Autodesk Inventor part; units mm, degrees
ref_plane "YZ Plane" through (0, 0, 0) normal (1, 0, 0) x (0, 1, 0)
ref_plane "XZ Plane" through (0, 0, 0) normal (0, 1, 0) x (-1, 0, 0)
ref_plane "XY Plane" through (0, 0, 0) normal (0, 0, 1) x (1, 0, 0)
sketch "Sketch1" plane through (0, 0, 0) normal (0, 1, 0) x (-1, 0, 0)
  circle A0 centre (0, 0) radius 26
  dimension "d0" = 52
extrude "Extrusion1" add sketch "Sketch1" along normal blind 7.2
chamfer "Chamfer2" distance 2 angle 45 1 edges at (26, 0, 0)
sketch "Sketch2" plane through (0, 7.2, 0) normal (0, 1, 0) x (1, 0, 0)
  line L0 (-13, -9.19) -> (23.96, -9.19)
  line L1 (23.96, -9.19) -> (23.96, 9.19)
  line L2 (23.96, 9.19) -> (-13, 9.19)
  line L3 (-13, 9.19) -> (-13, -9.19)
  point P0 (0, 0)
  dimension "d5" = 36.96
  dimension "d6" = 18.38
  dimension "d7" = 9.19
  dimension "d8" = 13
extrude "Extrusion2" cut sketch "Sketch2" against normal blind 4.6
sketch "Sketch3" plane through (23.96, 7.2, -9.19) normal (-1, 0, 0) x (0, 0, 1)
  line L0 (3.6, 0) -> (14.78, 0)
  line L1 (14.78, 0) -> (14.78, -3.2)
  line L2 (14.78, -3.2) -> (3.6, -3.2)
  line L3 (3.6, -3.2) -> (3.6, 0)
  line L4 (0, 0) -> (18.38, 0)
  line L5 (0, -4.6) -> (18.38, -4.6)
  line L6 (0, 0) -> (0, -4.6)
  line L7 (18.38, 0) -> (18.38, -4.6)
  point P0 (9.19, -7.2)
  dimension "d11" = 0
  dimension "d14" = 3.6
  dimension "d44" = 3.6
  dimension "d47" = 1.4
extrude "Extrusion3" cut sketch "Sketch3" against normal through all contours L0 L1 L2 L3
ref_plane "Work Plane1" through (-13, 7.2, 0) normal (0, 0, 1) x (1, 0, 0)
sketch "Sketch7" plane through (0, 2.6, 0) normal (0, 1, 0) x (1, 0, 0)
  line L0 (-13, 6.35) -> (22.56, 6.35)
  line L1 (22.56, 6.35) -> (22.56, -6.35)
  line L2 (22.56, -6.35) -> (-13, -6.35)
  line L3 (-13, -6.35) -> (-13, 6.35)
  line L4 (36.4, 0) -> (-36.4, 0)
  line L5 (-13, -9.19) -> (-13, 9.19)
  point P0 (0, 0)
  dimension "d28" = 12.7
  dimension "d29" = 35.56
  dimension "d30" = 6.35
  dimension "d31" = 0
extrude "Extrusion5" cut sketch "Sketch7" against normal blind 1.6
sketch "Sketch4" plane through (0, 7.2, 0) normal (0, 1, 0) x (1, 0, 0)
  circle A0 centre (-21, 0) radius 2.25
  arc A1 (25.392, 5.59) -> (25.392, -5.59) centre (0, 0) ccw
  point P0 (24.6995, 8.12)
  point P1 (24.6995, -8.12)
  dimension "d17" = 4.5
  dimension "d23" = 21
extrude "Extrusion4" cut sketch "Sketch4" against normal blind 5.2
fillet "Fillet4" radius 2.2 1 edges at (-23.25, 7.2, 0)
pattern_circular "Circular Pattern2" count 5 over 240 about axis through (0, 7.2, 0) along (0, 1, 0) of "Extrusion4", "Fillet4" both ways yes
chamfer "Chamfer3" distance 1.5 distance2 5 1 edges at (-13, 1, 0) measured on face at (-13, 5.6667, -2.1167)
equation "\"d44\" = d14"
equation "\"d30\" = 0.5 * d28"
equation "\"d24\" = 0.5 * d6"
properties part number "_3DPrint"
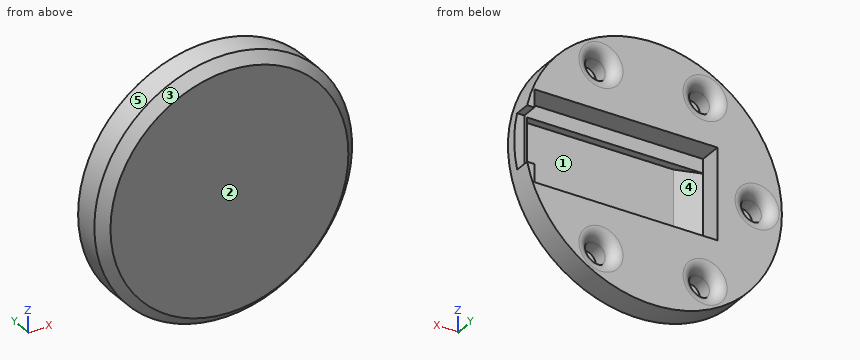
Can you work these out from the model? Positions are in its coordinate system, mm. Face numbers are marked on the shaded views. A direction names the side the tool comes from. Give positions to 0.01 mm unless a question says otherwise; leave off trailing zeros. Order: outer loops, then holes, each group sorted by start corner. A loop starts at its lowest first (then second) coordinate and runs counter-clockwise, first axis right, second up. Notation, with made-up numbers: M 53,4 L 63,4 A17 ccw 63,33 Z; hole C -34,-31.75 d3. An arc over 180 degrees is marked long. Write item = value, one per line. Start each with the question number.
Q1. I need wall thicknesses on probe 1 along X at (y, z) = (7, 17); probe 2 along Z at (x, y) = (10.5, 2.7); probe 3 along X at (y, z) = (4.75, -18). Which ranges of each line are inside material? Lowest first, please. Write a range as [from, to].
Q2. We'd pull the mould along X, two halves only. Please class the marked faces 1, 2 and 3: pulls with the +X half, pulls with the -X half, needs draft (parallel to the pull), parting line crosses it, or undercut.
Q3. Suppose I cut it at B-B (y = 6). Write out the boundary of the cut face in (x, z), plus the area to 3 significant figures.
Q4. For the marked faces 4 and 5, which set-ups out of +Z, -Z, +X, -X, +Y, -Y let a thin tool reach every point of the face, with its end or its side?
Q5. Suppose I cut it at A-A (z = 0). Write out the boundary of the cut face in (x, y), plus the area to 3 significant figures.
Q6. Will these pins go through, and if not, where does the flat tip stop? pin 1 Ø5 at (x, z) = (-9.5, 19) entering from +Y; pin 2 Ø1.5 at (x, z) = (-19, -0.5) entering from +Y; pin 3 Ø2 at (x, z) = (9, -2) entering from +Y; pin 4 Ø10 at (x, z) = (6.5, -6.5) entering from -Y.
Check result:
q1.probe_1 = [-19.67, -13.83], [-7.17, 7.17], [13.83, 19.67]
q1.probe_2 = [-23.79, -20.44], [-15.94, -9.19], [9.19, 15.94], [20.44, 23.79]
q1.probe_3 = [-18.76, -12.74], [-8.26, 8.26], [12.74, 18.76]
q2.face_1 = undercut
q2.face_2 = needs draft
q2.face_3 = parting line crosses it
q3.outline = M -13,-9.19 L -13,9.19 L 23.96,9.19 L 23.96,5.59 L 25.39,5.59 A26 ccw long 25.39,-5.59 L 23.96,-5.59 L 23.96,-9.19 Z; hole C -21,0 d4.98; hole C -10.5,-18.19 d4.98; hole C -10.5,18.19 d4.98; hole C 10.5,-18.19 d4.98; hole C 10.5,18.19 d4.98
q3.area = 1,330 mm2
q4.face_4 = +Y
q4.face_5 = +Y, -Y
q5.outline = M -26,2 L -24,0 L 24,0 L 26,2 L 26,4 L 23.96,4 L 23.96,2.6 L 22.56,2.6 L 22.56,1 L -8,1 L -13,2.5 L -13,7.2 L -16.55,7.2 A2.2 ccw -18.75,5 L -18.75,2 L -23.25,2 L -23.25,5 A2.2 ccw -25.45,7.2 L -26,7.2 Z
q5.area = 115 mm2
q6.pin_1 = 7.1
q6.pin_2 = 6.47
q6.pin_3 = 1
q6.pin_4 = 0
